```python
from build123d import *

# Parameters (mm, degrees)
F1_DEPTH = 5
F2_R     = 3
F3_DEPTH = 5
F4_R     = 3
F5_DEPTH = 5


with BuildPart() as f1:
    # F0 (on Top) → F1 (new body)
    with BuildSketch(Plane.XY):
        with BuildLine():
            ThreePointArc((0, 4), (-4, 0), (0, -4))
            Line((0, -4), (10, -4))
            ThreePointArc((10, -4), (14, 0), (10, 4))
            Line((10, 4), (0, 4))
        make_face()
    extrude(amount=F1_DEPTH)

    # F2 (on face) → F3 (join)
    with BuildSketch(Plane.XY.offset(5)):
        Circle(F2_R)
    extrude(amount=F3_DEPTH)

    # F4 (on face) → F5 (join)
    with BuildSketch(Plane(origin=(0, 0, 0), x_dir=(1, 0, 0), z_dir=(0, 0, -1))):
        with Locations((10, 0)):
            Circle(F4_R)
    extrude(amount=F5_DEPTH)


solid = f1.part
```
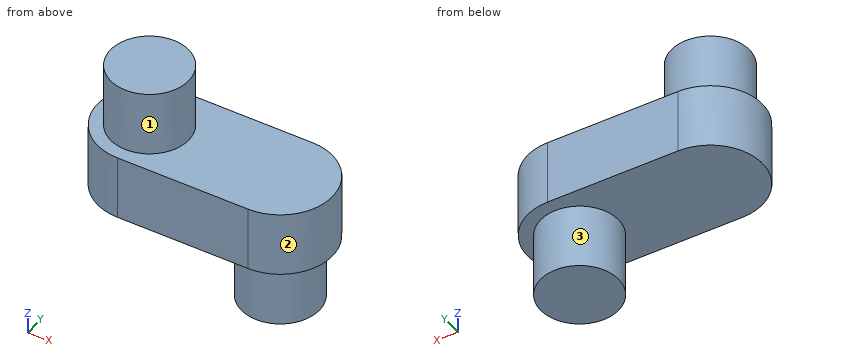
Here's how the part is built. I have some questions about the finished solid (model axes, mm). Face numbers are marked on the shaded views. A direction names the side the tool comes from. Give positions to 0.01 mm unless a question says otherwise; leave off trailing zeros. Write each loop counter-clockwise with the first axis right and the second up, starting at its lowest first coordinate (ties: lowest second). Pieces come first, ordered by that corner, then holes. Notation, with made-up numbers: (12, 21) -> (55, 21) arc R8 cw to (55, 32) -> close; hole circle Ø10 at (65.25, 27.5). An arc over 180 degrees is marked (long way). Use one line per item in the form item = value.
1) Suppose I cut it at C-C (z = -0.75). Please give me the cut outline in (x, y), and give its area (3 significant figures).
Verdict:
outline = circle Ø6 at (10, 0)
area = 28.3 mm2
2) Suppose I cut it at A-A (x = 12). Please give me the cut outline in (y, z), and give its area (3 significant figures).
Verdict:
outline = (-3.46, 0) -> (-2.24, 0) -> (-2.24, -5) -> (2.24, -5) -> (2.24, 0) -> (3.46, 0) -> (3.46, 5) -> (-3.46, 5) -> close
area = 57.0 mm2
3) Suppose I cut it at D-D (x = 2.75). Please give me the cut outline in (y, z).
Verdict:
outline = (-4, 0) -> (4, 0) -> (4, 5) -> (1.2, 5) -> (1.2, 10) -> (-1.2, 10) -> (-1.2, 5) -> (-4, 5) -> close
4) I'm going to push flat-ended pins straight in: pin 1 (1.5 mm diameter, centred on y = -2, z = -3.5, fed in from +X); pin 2 (4 mm diameter, centred on x = -2, y = 2.5, fed in from -Z); pin 3 (1 mm diameter, centred on y = -2, z = 0, fed in from +X). Where does each tip first touch, or does it pass through?
Verdict:
pin_1 = 12.73
pin_2 = 0
pin_3 = 13.71
5) If I drill on L1, parallel to Z at x = 1.75, y = 2.25; L2, parallel to Z at x = 2.5, y = -1.75; L3, parallel to X at y = 1, z = 6.25, over which ranges is the centre line in solid material (lowest first)? Write a range as [from, to].
Verdict:
L1 = [0, 10]
L2 = [0, 5]
L3 = [-2.83, 2.83]
6) Suppose I cut it at B-B (y = 0). Please give me the cut outline in (x, z), and give its area (3 significant figures).
Verdict:
outline = (-4, 0) -> (7, 0) -> (7, -5) -> (13, -5) -> (13, 0) -> (14, 0) -> (14, 5) -> (3, 5) -> (3, 10) -> (-3, 10) -> (-3, 5) -> (-4, 5) -> close
area = 150 mm2
7) On a 3-axis mill with a long thin cutter (end or side, diameter ignored), from which of +Z, -Z, +X, -X, +Y, -Y can I reach the whole of each face in a straight line? I mean the marked faces 1, 2 and 3. Say none if no direction works.
Verdict:
face_1 = +Z
face_2 = +Z, -Z, +X
face_3 = -Z
